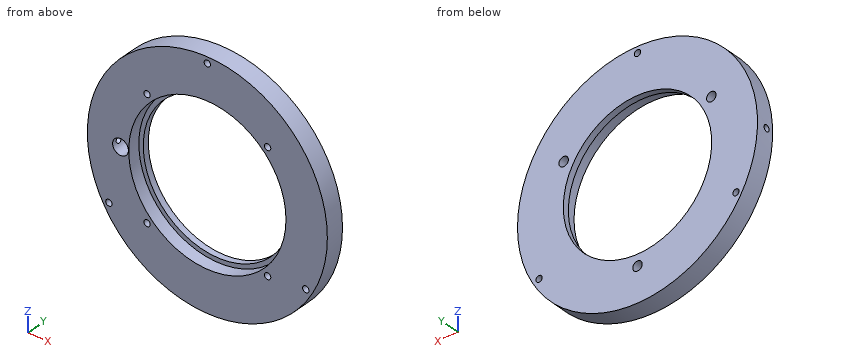
```python
from build123d import *

# Parameters (mm, degrees)
F0_R      = 38
F0_R_2    = 23.5
F1_DEPTH  = 6
F2_R      = 24.9
F3_DEPTH  = 4
F5_D      = 3
F5_DEPTH  = 5
F5_TIP    = 0.9012909285
F6_D      = 2
F8_D      = 2
F8_DEPTH  = 5
F8_TIP    = 0.600860619
F9_R      = 2.5
F10_DEPTH = 5
F13_D     = 2
F13_DEPTH = 10
F13_START = 2.0131603
F13_TIP   = 0.600860619


with BuildPart() as f1:
    # F0 (on Front) → F1 (new body)
    with BuildSketch(Plane.XZ):
        Circle(F0_R)
        Circle(F0_R_2, mode=Mode.SUBTRACT)
    extrude(amount=F1_DEPTH)

    # F2 (on face) → F3 (cut)
    with BuildSketch(Plane.XZ.offset(6)):
        Circle(F2_R)
    extrude(amount=-F3_DEPTH, mode=Mode.SUBTRACT)

    # F5
    with Locations(Plane(origin=(0, 0, 0), x_dir=(-1, 0, 0), z_dir=(0, 1, 0))):
        with Locations((23.3826859022, 13.5), (-23.3826859022, 13.5), (0, -27)):
            Hole(F5_D / 2, depth=F5_DEPTH)
            with Locations((0, 0, -(F5_DEPTH + F5_TIP / 2))):  # 118° drill point
                Cone(0, F5_D / 2, F5_TIP, mode=Mode.SUBTRACT)

    # F6 (through all)
    with Locations(Plane(origin=(0, 0, 0), x_dir=(-1, 0, 0), z_dir=(0, 1, 0))):
        with Locations((0, 36), (-31.1769145362, -18), (31.1769145362, -18)):
            Hole(F6_D / 2)

    # F8
    with Locations(Plane.XZ.offset(6)):
        with Locations((-19.091883092, 19.091883092), (-19.091883092, -19.091883092), (19.091883092, -19.091883092), (19.091883092, 19.091883092)):
            Hole(F8_D / 2, depth=F8_DEPTH)
            with Locations((0, 0, -(F8_DEPTH + F8_TIP / 2))):  # 118° drill point
                Cone(0, F8_D / 2, F8_TIP, mode=Mode.SUBTRACT)

    # F9 (on face) → F10 (cut)
    with BuildSketch(Plane.XZ.offset(6)):
        with Locations((-27.5, 0)):
            Circle(F9_R)
    extrude(amount=-F10_DEPTH, mode=Mode.SUBTRACT)

    # F13
    # its depths count from where the whole tool has entered the part; down to there all is cleared
    with Locations(Plane(origin=(-40, 0, 0), x_dir=(0, 1, 0), z_dir=(-1, 0, 0)).offset(-F13_START)):
        with Locations((-3.6, 0)):
            Hole(F13_D / 2, depth=F13_DEPTH)
            with Locations((0, 0, -(F13_DEPTH + F13_TIP / 2))):  # 118° drill point
                Cone(0, F13_D / 2, F13_TIP, mode=Mode.SUBTRACT)


solid = f1.part
```
Work out the finished part from the listing and answer in its coordinate system (mm). Give positions to 0.01 mm unless a question says otherwise; leave off trailing zeros. Loops run counter-clockwise (first coordinate to the right, second up) from the corner with the lowest first, then second, coordinate; pieces in that order, holes last. Notation, with made-up numbers: (-29.5, -4) -> (25.5, -4) arc R22 ccw to (25.5, 5) -> close; hole circle Ø1 at (19.5, 36). An arc over 180 degrees is marked (long way). Put each result on its own line as item: value. Start each with the question number.
Item 1: The part is cut by section B-B (x = 9.5). Give the vertices of the cut face in (y, z).
Item 2: The part is cut by section A-A (z = 0). Give the vertices of the cut face in (x, y), then the cut area to 3 significant figures.
Item 3: The part is cut by section C-C (z = -15.5). Give the vertices of the cut face in (x, y).
Item 4: The part is cut by section D-D (y = -3.5). State how many separate pieces and enclosed holes the cut face has, then the cut area to 3 significant figures.
Item 5: Each of these flat-tipped pins is pushed along its axis until it touches: P1, Ø2, axis at y = -4, z = -11, coming from the +X side; P2, Ø1, axis at y = -4.5, z = 12, coming from the -X side; P3, Ø1, axis at x = -12.5, y = -2.5, coming from the -Z side. Where does it stop, or does it pass through?
Item 6: Find the intervals of material crossed by L1, parallel to X at y = -1, z = -27.5; L2, parallel to Z at x = 13.5, y = -3.75; L3, parallel to X at y = -2.7, z = 13.5, in increasing order. Write a range as [from, to].
Answers below:
1. outline: (-6, -36.79) -> (0, -36.79) -> (0, -21.49) -> (-2, -21.49) -> (-2, -23.02) -> (-6, -23.02) -> close; (-6, 23.02) -> (-2, 23.02) -> (-2, 21.49) -> (0, 21.49) -> (0, 36.79) -> (-6, 36.79) -> close
2. outline: (-38, -6) -> (-30, -6) -> (-30, -4.6) -> (-38, -4.6) -> close; (-38, -2.6) -> (-30, -2.6) -> (-30, -1) -> (-25, -1) -> (-25, -6) -> (-24.9, -6) -> (-24.9, -2) -> (-23.5, -2) -> (-23.5, 0) -> (-38, 0) -> close; (23.5, -2) -> (24.9, -2) -> (24.9, -6) -> (38, -6) -> (38, 0) -> (23.5, 0) -> close
2. area: 122 mm2
3. outline: (-34.7, -6) -> (-19.49, -6) -> (-19.49, -2) -> (-17.66, -2) -> (-17.66, 0) -> (-34.7, 0) -> close; (17.66, -2) -> (19.49, -2) -> (19.49, -6) -> (34.7, -6) -> (34.7, 0) -> (17.66, 0) -> close
4. separate pieces: 1
4. enclosed holes: 11
4. area: 2,510 mm2
5. P1: x = 36.66
5. P2: x = -36.22
5. P3: z = -36.06
6. L1: [-26.22, -1.41], [1.41, 26.22]
6. L2: [-35.52, -20.92], [20.92, 35.52]
6. L3: [-35.52, -24.88], [-21.88, -20.92], [20.92, 21.88], [24.88, 35.52]
